from build123d import *

# Parameters (mm, degrees)
F0_W     = 80
F0_H     = 80
F1_DEPTH = 80
F2_R     = 15
F3_DEPTH = 80.001
F4_R     = 5


with BuildPart() as f1:
    # F0 (on Top) → F1 (new body)
    with BuildSketch(Plane.XY):
        with Locations((20.5740025267, -1.6444633871)):
            Rectangle(F0_W, F0_H)
    extrude(amount=F1_DEPTH)

    # F2 (on face) → F3 (cut, through all)
    with BuildSketch(Plane.XY.offset(80)):
        with Locations((17.8592021294, 0)):
            Circle(F2_R)
    extrude(amount=-F3_DEPTH, mode=Mode.SUBTRACT)

    # F4
    f4_edges = [f1.edges().sort_by_distance(p)[0] for p in [
        (20.574003, 38.355537, 0),
        (60.574003, -1.644463, 0),
        (20.574003, -41.644463, 0),
        (-19.425997, -1.644463, 0),
        (60.574003, -1.644463, 80),
        (60.574003, -41.644463, 40),
        (60.574003, 38.355537, 40),
        (20.574003, 38.355537, 80),
        (-19.425997, -1.644463, 80),
        (20.574003, -41.644463, 80),
        (2.859202, 0, 80),
        (-19.425997, 38.355537, 40),
    ]]
    fillet(f4_edges, radius=F4_R)


solid = f1.part
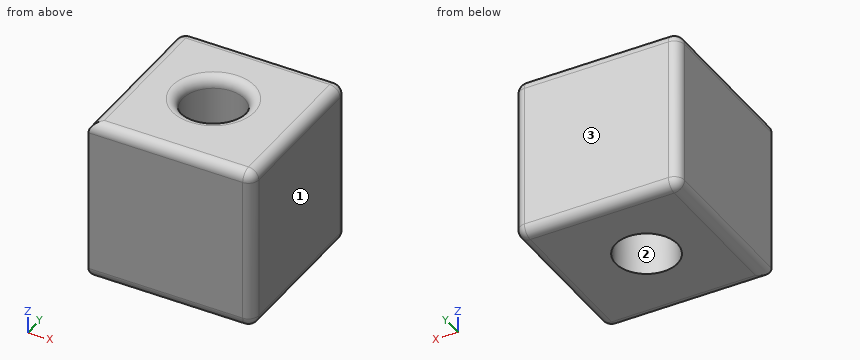
Read the model definition and answer for the solid it produces. Units are mm, in the model's axes. Face numbers are marked on the shaded views. Coordinates: 2 decimals unless noted, no trailing zeros. Write each loop counter-clockwise with the first axis right and the second up, starting at its lowest first coordinate (ties: lowest second). Pieces come first, ordered by that corner, then holes. Notation, with made-up numbers: M -38,54.5 L 2,54.5 A16 cw 2,71.5 Z; hole C 3.5,71 d2. An arc over 180 degrees is marked long. Use a Markdown table: item, result.
Q1. The part is cut by section A-A, the plane y = 0. Write down the section's boundary in (x, z), then the cut area to 3 significant figures.
Answer block:
| item | result |
|---|---|
| outline | M -19.43,5 A5 ccw -14.43,0 L 2.86,0 L 2.86,75 A5 ccw -2.14,80 L -14.43,80 A5 ccw -19.43,75 Z; M 32.86,0 L 55.57,0 A5 ccw 60.57,5 L 60.57,75 A5 ccw 55.57,80 L 37.86,80 A5 ccw 32.86,75 Z |
| area | 3,970 mm2 |
Q2. Straight lines are drawn through the part: L1, parallel to X at y = -0.5, z = 20.5; L2, parallel to Y at x = 15, z = 47; L3, parallel to Y at x = 30, z = 51. For each, find the intervals that lie inside material, in ascending order. Write a range as [from, to].
Answer block:
| item | result |
|---|---|
| L1 | x = [-19.43, 2.87], [32.85, 60.57] |
| L2 | y = [-41.64, -14.72], [14.72, 38.36] |
| L3 | y = [-41.64, -8.81], [8.81, 38.36] |
Q3. This flat-tipped pin is pushed along its axis until it touches: pin 1 Ø24 at (x, y) = (17.86, 0) entering from +Z. Where does it stop, or does it pass through?
Answer block:
| item | result |
|---|---|
| pin 1 | passes through |
Q4. The part is cut by section B-B, the plane z = 50. Write down the section's boundary in (x, y), then the cut area to 3 significant figures.
Answer block:
| item | result |
|---|---|
| outline | M -19.43,-41.64 L 55.57,-41.64 A5 ccw 60.57,-36.64 L 60.57,33.36 A5 ccw 55.57,38.36 L -14.43,38.36 A5 ccw -19.43,33.36 Z; hole C 17.86,0 d30 |
| area | 5,680 mm2 |
Q5. Determine the mould class of the marked faces 1, 2 and 3 for opening direction Y: released by +Y, released by -Y, zero draft, split by the parting line, or undercut.
Answer block:
| item | result |
|---|---|
| face 1 | zero draft |
| face 2 | undercut |
| face 3 | released by +Y |
